Part print with two shaded views. Sizes in mm from the minimum x, y, z corner. Coordinates: 2 decimals unless noted, no trailing zeros. Order: outer loops, then holes, each group sorted by start corner. A loop starts at its lowest first (then second) coordinate and runs counter-clockwise, first axis right, second up.
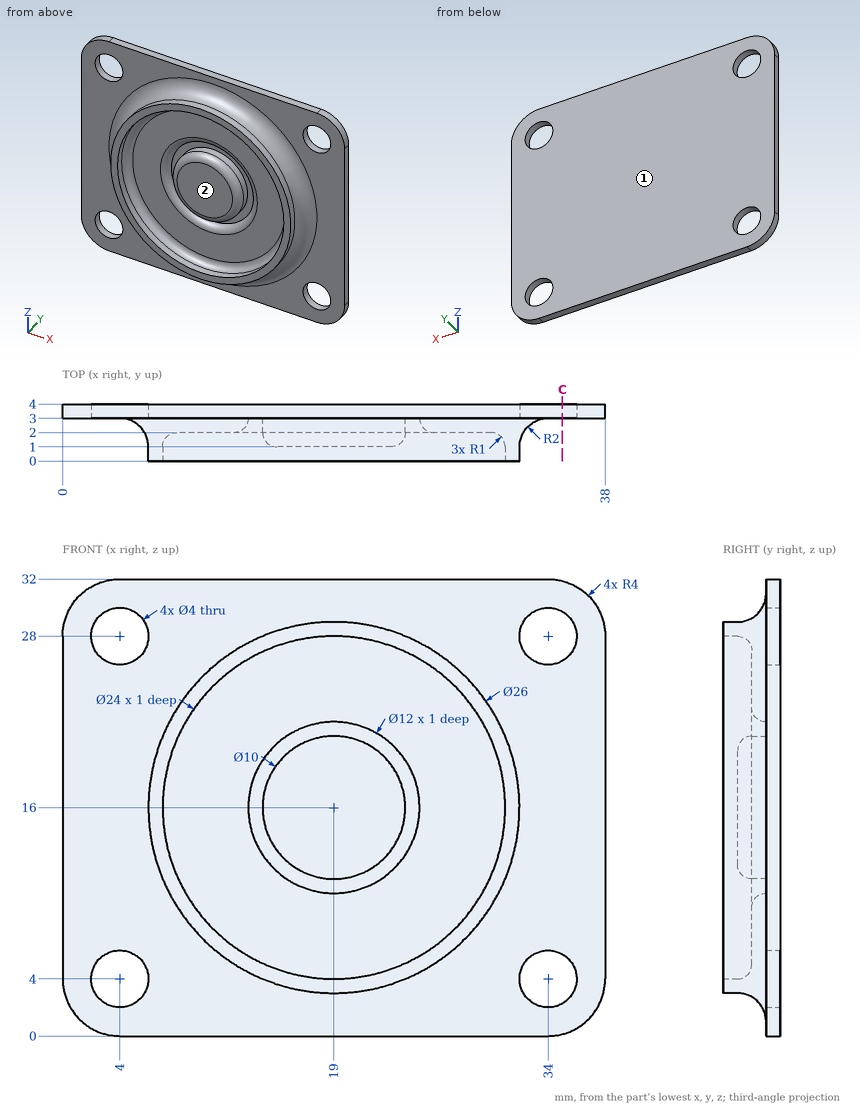
Q1. Wall check: line 1 along X through (y, z) = (3.4, 28); line 2 along X through (y, z) = (0.65, 16); line 3 along Y through (x, z) = (13.5, 7). Give the ranges that are in metal, low to high.
Results list:
line 1: x = 0 to 2, 6 to 32, 36 to 38
line 2: x = 6 to 7, 31 to 32
line 3: y = 2 to 4
Q2. Mould opens along X. For the marked faces 1 and 2 say: pulls with the +X half, pulls with the -X half, needs draft (parallel to the pull), parting line crosses it, or undercut.
Results list:
face 1: needs draft
face 2: undercut
Q3. Pin check, flat tips, straight feed: pin 1 Ø6 at (x, z) = (17, 17) entering from -Y; pin 2 Ø1 at (y, z) = (1, 4.5) entering from -X; pin 3 Ø4 at (x, z) = (7.5, 8) entering from -Y; pin 4 Ø4.5 at (x, z) = (4, 28) entering from -Y. Stop position of each tip, or through.
Results list:
pin 1: stops at y = 1
pin 2: stops at x = 12.07
pin 3: stops at y = 0
pin 4: stops at y = 3
Q4. Cut at C-C on x = 35. Write the cut outline in (y, z), and give its area (3 significant figures).
Results list:
outline: (3, 0.13) - (4, 0.13) - (4, 2.27) - (3, 2.27) - close; (3, 5.73) - (4, 5.73) - (4, 26.27) - (3, 26.27) - close; (3, 29.73) - (4, 29.73) - (4, 31.87) - (3, 31.87) - close
area: 24.8 mm2
